```python
from build123d import *

# Parameters (mm, degrees)
BOSS_EXTRUDE1_DEPTH = 7
FILLET1_R           = 8.5
FILLET2_R           = 5.5
FILLET3_R           = 13.5
SKETCH3_W           = 27
SKETCH3_H           = 13.5
CUT_EXTRUDE1_DEPTH  = 1.8
BOSS_EXTRUDE2_DEPTH = 5
BOSS_EXTRUDE3_DEPTH = 7
SKETCH10_R          = 2.5
CUT_EXTRUDE3_DEPTH  = 21
CUT_EXTRUDE5_REACH  = 41.994
SKETCH12_W          = 12
SKETCH12_H          = 13.5
CUT_EXTRUDE6_REACH  = 39.182
SKETCH13_R          = 1
SKETCH17_R          = 2
CUT_EXTRUDE14_DEPTH = 4
FILLET4_R           = 3
CUT_EXTRUDE16_REACH = 42.725
SKETCH19_W          = 12
SKETCH19_H          = 4.5
CHAMFER5_SIZE       = 3
CHAMFER5_SIZE2      = 5.196152423
CUT_EXTRUDE17_DEPTH = 4
SHELL1_START        = 3
SHELL1_DEPTH        = 4
SHELL1_START_2      = -9
SHELL1_2_OUTLINE_R  = 5.5
SHELL1_2_DEPTH      = 1
SHELL1_START_3      = 4.8
SHELL1_3_DEPTH      = 2.2
SKETCH21_R          = 4.3
CUT_EXTRUDE18_DEPTH = 5
FILLET5_R           = 9.5
FILLET6_R           = 2.5


# Read off the part's stored shape, not the designer's step: Shell1
with BuildPart() as part:
    # Sketch2 → Boss-Extrude1 (new body)
    with BuildSketch(Plane(origin=(0, 0, 0), x_dir=(0, 0, -1), z_dir=(1, 0, 0))):
        Polygon((-13.5, -17.5), (13.5, -17.5), (13.5, 17.5), (5.5, 32.5), (-5.5, 32.5), (-13.5, 17.5), align=None)
    extrude(amount=BOSS_EXTRUDE1_DEPTH)

    # Fillet1
    fillet1_edges = [part.edges().sort_by_distance(p)[0] for p in [
        (3.5, 32.5, 5.5),
        (3.5, 32.5, -5.5),
    ]]
    fillet(fillet1_edges, radius=FILLET1_R)

    # Fillet2
    fillet2_edges = [part.edges().sort_by_distance(p)[0] for p in [
        (3.5, 17.5, -13.5),
        (3.5, 17.5, 13.5),
    ]]
    fillet(fillet2_edges, radius=FILLET2_R)

    # Fillet3
    fillet3_edges = [part.edges().sort_by_distance(p)[0] for p in [
        (3.5, -17.5, 13.5),
        (3.5, -17.5, -13.5),
    ]]
    fillet(fillet3_edges, radius=FILLET3_R - 0.0001)  # a hair under: the kernel refuses the full size

    # Sketch3 → Cut-Extrude1 (cut)
    with BuildSketch(Plane.ZY):
        with Locations((0, -10.75)):
            Rectangle(SKETCH3_W, SKETCH3_H)
    extrude(amount=-CUT_EXTRUDE1_DEPTH, mode=Mode.SUBTRACT)

    # Sketch6 → Boss-Extrude2 (add)
    with BuildSketch(Plane.ZY):
        with BuildLine():
            Line((-13.5, 14), (13.5, 14))
            Line((13.5, 14), (13.5, 16.125))
            ThreePointArc((13.5, 16.125), (13.293303509, 17.618632471), (12.688749833, 19))
            Line((12.688749833, 19), (-12.688749833, 19))
            ThreePointArc((-12.688749833, 19), (-13.293303509, 17.618632471), (-13.5, 16.125))
            Line((-13.5, 16.125), (-13.5, 14))
        make_face()
    extrude(amount=BOSS_EXTRUDE2_DEPTH)

    # Sketch9 → Boss-Extrude3 (add)
    with BuildSketch(Plane.ZY.offset(5)):
        with BuildLine():
            Line((-13.5, 14), (-13.5, -4))
            Line((-13.5, -4), (13.5, -4))
            Line((13.5, -4), (13.5, 14))
            Line((13.5, 14), (13.5, 16.125))
            ThreePointArc((13.5, 16.125), (13.293303509, 17.618632471), (12.688749833, 19))
            Line((12.688749833, 19), (-12.688749833, 19))
            ThreePointArc((-12.688749833, 19), (-13.293303509, 17.618632471), (-13.5, 16.125))
            Line((-13.5, 16.125), (-13.5, 14))
        make_face()
    extrude(amount=BOSS_EXTRUDE3_DEPTH)

    # Sketch10 → Cut-Extrude3 (cut)
    with BuildSketch(Plane(origin=(7, 0, 0), x_dir=(0, 0, -1), z_dir=(1, 0, 0))):
        with Locations((0, 4.75)):
            Circle(SKETCH10_R)
    extrude(amount=-CUT_EXTRUDE3_DEPTH, mode=Mode.SUBTRACT)

    # Sketch12 → Cut-Extrude5 (cut, up to next)
    with BuildSketch(Plane(origin=(7, 0, 0), x_dir=(0, 0, -1), z_dir=(1, 0, 0)), mode=Mode.PRIVATE) as cut_extrude5_sk1:
        with Locations((0, -10.75)):
            Rectangle(SKETCH12_W, SKETCH12_H)
    cut_extrude5_tool1 = extrude(cut_extrude5_sk1.sketch, amount=-CUT_EXTRUDE5_REACH, mode=Mode.PRIVATE) & part.part
    add(cut_extrude5_tool1.solids().sort_by_distance((7, -10.75, 0))[0], mode=Mode.SUBTRACT)

    # Sketch13 → Cut-Extrude6 (cut, up to next)
    with BuildSketch(Plane.ZY, mode=Mode.PRIVATE) as cut_extrude6_sk1:
        with Locations((-7.5, 23.5)):
            Circle(SKETCH13_R)
    cut_extrude6_tool1 = extrude(cut_extrude6_sk1.sketch, amount=-CUT_EXTRUDE6_REACH, mode=Mode.PRIVATE) & part.part
    # Sketch13 → Cut-Extrude6 (cut, up to next)
    with BuildSketch(Plane.ZY, mode=Mode.PRIVATE) as cut_extrude6_sk2:
        with Locations((-10, -8.5)):
            Circle(SKETCH13_R)
    cut_extrude6_tool2 = extrude(cut_extrude6_sk2.sketch, amount=-CUT_EXTRUDE6_REACH, mode=Mode.PRIVATE) & part.part
    # Sketch13 → Cut-Extrude6 (cut, up to next)
    with BuildSketch(Plane.ZY, mode=Mode.PRIVATE) as cut_extrude6_sk3:
        with Locations((10, -8.5)):
            Circle(SKETCH13_R)
    cut_extrude6_tool3 = extrude(cut_extrude6_sk3.sketch, amount=-CUT_EXTRUDE6_REACH, mode=Mode.PRIVATE) & part.part
    # Sketch13 → Cut-Extrude6 (cut, up to next)
    with BuildSketch(Plane.ZY, mode=Mode.PRIVATE) as cut_extrude6_sk4:
        with Locations((7.5, 23.5)):
            Circle(SKETCH13_R)
    cut_extrude6_tool4 = extrude(cut_extrude6_sk4.sketch, amount=-CUT_EXTRUDE6_REACH, mode=Mode.PRIVATE) & part.part
    add(cut_extrude6_tool1.solids().sort_by_distance((0, 23.5, -7.5))[0], mode=Mode.SUBTRACT)
    add(cut_extrude6_tool2.solids().sort_by_distance((0, -8.5, -10))[0], mode=Mode.SUBTRACT)
    add(cut_extrude6_tool3.solids().sort_by_distance((0, -8.5, 10))[0], mode=Mode.SUBTRACT)
    add(cut_extrude6_tool4.solids().sort_by_distance((0, 23.5, 7.5))[0], mode=Mode.SUBTRACT)

    # Sketch17 → Cut-Extrude14 (cut)
    with BuildSketch(Plane.ZY):
        with Locations((-7.5, 23.5)):
            Circle(SKETCH17_R)
        with Locations((7.5, 23.5)):
            Circle(SKETCH17_R)
        with Locations((-10, -8.5)):
            Circle(SKETCH17_R)
        with Locations((10, -8.5)):
            Circle(SKETCH17_R)
    extrude(amount=-CUT_EXTRUDE14_DEPTH, mode=Mode.SUBTRACT)

    # Fillet4
    fillet4_edges = [part.edges().sort_by_distance(p)[0] for p in [
        (4.4, -16.093424605, -6),
        (4.4, -16.093424605, 6),
    ]]
    fillet(fillet4_edges, radius=FILLET4_R)

    # Sketch19 → Cut-Extrude16 (cut, up to next)
    with BuildSketch(Plane.XZ.offset(4), mode=Mode.PRIVATE) as cut_extrude16_sk1:
        with Locations((-6, -11.25)):
            Rectangle(SKETCH19_W, SKETCH19_H)
    cut_extrude16_tool1 = extrude(cut_extrude16_sk1.sketch, amount=-CUT_EXTRUDE16_REACH, mode=Mode.PRIVATE) & part.part
    # Sketch19 → Cut-Extrude16 (cut, up to next)
    with BuildSketch(Plane.XZ.offset(4), mode=Mode.PRIVATE) as cut_extrude16_sk2:
        with Locations((-6, 11.25)):
            Rectangle(SKETCH19_W, SKETCH19_H)
    cut_extrude16_tool2 = extrude(cut_extrude16_sk2.sketch, amount=-CUT_EXTRUDE16_REACH, mode=Mode.PRIVATE) & part.part
    add(cut_extrude16_tool1.solids().sort_by_distance((-6, -4, -11.25))[0], mode=Mode.SUBTRACT)
    add(cut_extrude16_tool2.solids().sort_by_distance((-6, -4, 11.25))[0], mode=Mode.SUBTRACT)

    # Chamfer5
    chamfer5_edges = [part.edges().sort_by_distance(p)[0] for p in [
        (-8.5, -4, -9),
        (-8.5, -4, 9),
    ]]
    chamfer5_side = [part.faces().sort_by_distance(p)[0] for p in [
        (-8.5, -4, 0),
    ]]
    chamfer(chamfer5_edges, length=CHAMFER5_SIZE, length2=CHAMFER5_SIZE2, reference=chamfer5_side[0])

    # Sketch20 → Cut-Extrude17 (cut)
    with BuildSketch(Plane(origin=(7, 0, 0), x_dir=(0, 0, -1), z_dir=(1, 0, 0))):
        Polygon((2.309401077, 8.75), (-2.309401077, 8.75), (-4.618802154, 4.75), (-2.309401077, 0.75), (2.309401077, 0.75), (4.618802154, 4.75), align=None)
    extrude(amount=-CUT_EXTRUDE17_DEPTH, mode=Mode.SUBTRACT)

    # Shell1 outline → Shell1 (cut)
    with BuildSketch(Plane.YZ.offset(SHELL1_START)):
        with BuildLine():
            Line((4.75, 8.082903769), (11.75, 4.041451884))
            Line((11.75, 4.041451884), (11.75, -4.041451884))
            Line((11.75, -4.041451884), (4.75, -8.082903769))
            Line((4.75, -8.082903769), (-1, -4.763139721))
            Line((-1, -4.763139721), (-1, -10.5))
            Line((-1, -10.5), (16.125, -10.5))
            ThreePointArc((16.125, -10.5), (16.731339062, -10.42535625), (17.301470588, -10.205882353))
            Line((17.301470588, -10.205882353), (18.863900358, -9.372586476))
            ThreePointArc((18.863900358, -9.372586476), (21.090892464, -3.118653074), (27.564772739, -4.588364277))
            ThreePointArc((27.564772739, -4.588364277), (28.99280733, -2.706918934), (29.5, -0.4))
            Line((29.5, -0.4), (29.5, 0.4))
            ThreePointArc((29.5, 0.4), (28.99280733, 2.706918934), (27.564772739, 4.588364277))
            ThreePointArc((27.564772739, 4.588364277), (21.090892464, 3.118653074), (18.863900358, 9.372586476))
            Line((18.863900358, 9.372586476), (17.301470588, 10.205882353))
            ThreePointArc((17.301470588, 10.205882353), (16.731339062, 10.42535625), (16.125, 10.5))
            Line((16.125, 10.5), (-1, 10.5))
            Line((-1, 10.5), (-1, 4.763139721))
            Line((-1, 4.763139721), (4.75, 8.082903769))
        make_face()
    extrude(amount=SHELL1_DEPTH, mode=Mode.SUBTRACT)

    # Shell1 2 outline → Shell1 2 (cut)
    with BuildSketch(Plane.YZ.offset(SHELL1_START_2)):
        Polygon((16, -6), (16, 6), (2, 6), (-1, 4.267949192), (-1, -4.267949192), (2, -6), align=None)
        with Locations((4.75, 0)):
            Circle(SHELL1_2_OUTLINE_R, mode=Mode.SUBTRACT)
    extrude(amount=SHELL1_2_DEPTH, mode=Mode.SUBTRACT)

    # Shell1 3 outline → Shell1 3 (cut)
    with BuildSketch(Plane.YZ.offset(SHELL1_START_3)):
        with BuildLine():
            Line((-1, -10.5), (-1, -9))
            Line((-1, -9), (-3.601020514, -9))
            ThreePointArc((-3.601020514, -9), (-3.506398333, -9.747131669), (-3.525062814, -10.5))
            Line((-3.525062814, -10.5), (-1, -10.5))
        make_face()
        with BuildLine():
            Line((-3.601020514, 9), (-1, 9))
            Line((-1, 9), (-1, 10.5))
            Line((-1, 10.5), (-3.525062814, 10.5))
            ThreePointArc((-3.525062814, 10.5), (-3.506398333, 9.747131669), (-3.601020514, 9))
        make_face()
    extrude(amount=SHELL1_3_DEPTH, mode=Mode.SUBTRACT)

    # Sketch21 → Cut-Extrude18 (cut)
    with BuildSketch(Plane.ZY.offset(12)):
        with Locations((0, 4.75)):
            Circle(SKETCH21_R)
    extrude(amount=-CUT_EXTRUDE18_DEPTH, mode=Mode.SUBTRACT)

    # Fillet5
    fillet5_edges = [part.edges().sort_by_distance(p)[0] for p in [
        (-12, 19, 0),
    ]]
    fillet(fillet5_edges, radius=FILLET5_R)

    # Fillet6
    fillet6_edges = [part.edges().sort_by_distance(p)[0] for p in [
        (0, 19, 0),
    ]]
    fillet(fillet6_edges, radius=FILLET6_R - 0.0001)  # a hair under: the kernel refuses the full size


solid = part.part
```
Can you work these out from the model? Positions are in its coordinate system, mm. A direction names the side the tool comes from. Coordinates: 2 decimals unless noted, no trailing zeros. Write each loop counter-clockwise with the first axis right and the second up, starting at its lowest first coordinate (ties: lowest second). Pieces come first, ordered by that corner, then holes. Notation, with made-up numbers: (-1.75, 52.5) - (7.25, 52.5) arc R21 ccw to (7.25, 63.5) - close; hole circle Ø6 at (37, -28). An arc over 180 degrees is marked (long way). Return JSON: item names as keys, results as strings.
Q1. I'm going to push flat-ended pins straight in: pin 1 Ø0.5 at (x, y) = (-8.5, 5.5) entering from +Z; pin 2 Ø3.5 at (x, z) = (-8, -1) entering from -Y; pin 3 Ø6.5 at (y, z) = (4.75, 0) entering from +X. Where does each tip first touch, or does it pass through?
Computed values:
{"pin 1": "stops at z = 9", "pin 2": "stops at y = -4", "pin 3": "stops at x = 3"}
Q2. Please list where these lines run through material, in increasing order: L1, parallel to X at y = 5, z = -5.75; L2, parallel to Y at x = 6.25, z = -7.5; L3, parallel to X at y = 0, z = -0.5. Write a range as from..to.
Computed values:
{"L1": "x = -12..-9, -8..-5, 0..7", "L2": "y = -12.01..-1, 3.74..5.76, 18.5..22.5, 24.5..28.67", "L3": "x = -12..-5, 0..7"}
Q3. If we section it at C-C (y = -8.5): Please give me the cut outline in (x, z).
Computed values:
{"outline": "(1.8, -12.73) - (7, -12.73) - (7, -11) - (4, -11) - (4, -12) - (1.8, -12) - close; (1.8, -8) - (4, -8) - (4, -9) - (7, -9) - (7, -6) - (1.8, -6) - close; (1.8, 6) - (7, 6) - (7, 9) - (4, 9) - (4, 8) - (1.8, 8) - close; (1.8, 12) - (4, 12) - (4, 11) - (7, 11) - (7, 12.73) - (1.8, 12.73) - close"}
Q4. Thinking about a two-plate mould opening in Y: for faces 4 (the flat face through (4, -7, 6)), 5 (the flat face through (-8.5, -1.4, 7.5)), 6 (the flat face through (-8.507, 0.479, -5.122)), 7 (the flat face through (4.972, 18.072, -9.795)), which applies, +Y half, -Y half, draft (parallel to the pull), parting line (faces both ways), or undercut?
Computed values:
{"face 4": "draft", "face 5": "-Y half", "face 6": "undercut", "face 7": "undercut"}
Q5. If we section it at B-B (x = 0.5): Please give me the cut outline in (y, z) (3 decimals).
Computed values:
{"outline": "(-4, -13.5) - (16.125, -13.5) arc R5.5 ccw to (18.713, -12.853) - (28, -7.9) arc R8.5 ccw to (32.5, -0.4) - (32.5, 0.4) arc R8.5 ccw to (28, 7.9) - (18.713, 12.853) arc R5.5 ccw to (16.125, 13.5) - (-4, 13.5) - close; hole circle Ø5 at (4.75, 0); hole circle Ø4 at (23.5, -7.5); hole circle Ø4 at (23.5, 7.5)"}
Q6. If we section it at A-A (y = 23.5): Please give me the cut outline in (x, z), then the cut area to 3 significant figures.
Computed values:
{"outline": "(0, -10.3) - (7, -10.3) - (7, -8.5) - (4, -8.5) - (4, -9.5) - (0, -9.5) - close; (0, -5.5) - (4, -5.5) - (4, -6.5) - (7, -6.5) - (7, -2.5) - (3, -2.5) - (3, 2.5) - (7, 2.5) - (7, 6.5) - (4, 6.5) - (4, 5.5) - (0, 5.5) - close; (0, 9.5) - (4, 9.5) - (4, 8.5) - (7, 8.5) - (7, 10.3) - (0, 10.3) - close", "area": "80.2 mm2"}
Q7. On a 3-axis mill with a long thin cutter (end or side, diameter ignored), from which of +Z, -Z, +X, -X, +Y, -Y can I reach the whole of each face in a straight line? I mean faces 1 (the flat face through (4, 22.6, 8.4)), 2 (the flat face through (5.028, 6.778, 3.448)), 3 (the flat face through (-8.507, 0.521, 5.146)). Say none if no direction works.
Computed values:
{"face 1": "-X", "face 2": "+X", "face 3": "none"}
Q8. If we section it at D-D (y = -1.5): Please give me the cut outline in (x, z).
Computed values:
{"outline": "(-12, -7.44) - (-5, -7.44) - (-5, 7.44) - (-12, 7.44) - close; (0, -13.5) - (7, -13.5) - (7, -10.5) - (4.8, -10.5) - (4.8, -9) - (7, -9) - (7, 9) - (4.8, 9) - (4.8, 10.5) - (7, 10.5) - (7, 13.5) - (0, 13.5) - close"}
